Work out the finished part from the listing and answer in its coordinate system (mm). Face numbers are marked on the shaded views. A direction names the side the tool comes from. Round coordinates to 2 decimals unless told otherwise and drop trailing zeros. Loops run counter-clockwise (first coordinate to the right, second up) from the corner with the lowest first, then second, coordinate; pieces in that order, holes last.
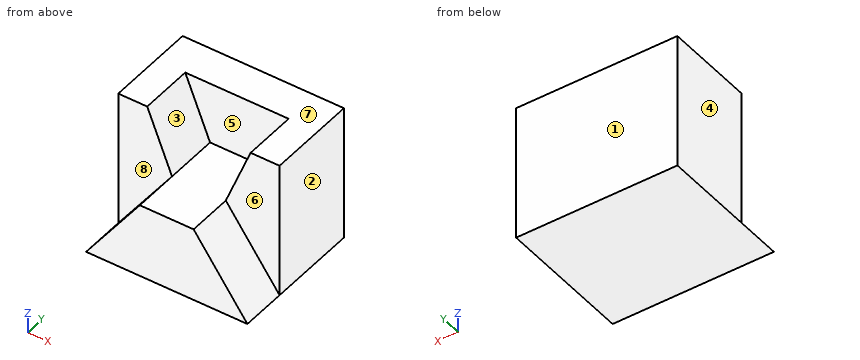
```python
from build123d import *

# Parameters (mm, degrees)
F1_DEPTH = 33
F2_DEPTH = 11
F3_DEPTH = 24


with BuildPart() as f1:
    # F0 (on Front) → F1 (new body)
    with BuildSketch(Plane.XZ):
        Polygon((13, 18), (0, 0), (39, 0), (26, 18), align=None)
        Polygon((0, 33), (0, 0), (13, 18), (7, 33), align=None)
        Polygon((26, 18), (39, 0), (39, 33), (32, 33), align=None)
        Polygon((7, 33), (13, 18), (26, 18), (32, 33), align=None)
    extrude(amount=-F1_DEPTH)

    # F0 (on Front) → F2 (cut)
    with BuildSketch(Plane.XZ):
        Polygon((0, 33), (0, 0), (13, 18), (7, 33), align=None)
        Polygon((7, 33), (13, 18), (26, 18), (32, 33), align=None)
        Polygon((26, 18), (39, 0), (39, 33), (32, 33), align=None)
    extrude(amount=-F2_DEPTH, mode=Mode.SUBTRACT)

    # F0 (on Front) → F3 (cut)
    with BuildSketch(Plane.XZ):
        Polygon((7, 33), (13, 18), (26, 18), (32, 33), align=None)
    extrude(amount=-F3_DEPTH, mode=Mode.SUBTRACT)


solid = f1.part
```
1. Find section C-C (x = 22.5). Write down the section's boundary in (y, z).
Answer key:
outline: (0, 0) - (33, 0) - (33, 33) - (24, 33) - (24, 18) - (0, 18) - close
2. Consider probe 1 along Y at (x, z) = (6, 11); probe 2 along Y at (x, z) = (24.5, 26); probe 3 along X at (y, z) = (23, 23.5). Determine where each line is inside the solid, lowest interval first.
Answer key:
probe 1: y = 11 to 33
probe 2: y = 24 to 33
probe 3: x = 0 to 10.8, 28.2 to 39
3. Determine the mould class of the marked faces 1, 2 and 3 for opening direction X: +X half, -X half, draft (parallel to the pull), parting line (faces both ways), or undercut.
Answer key:
face 1: draft
face 2: +X half
face 3: undercut
4. Find section B-B (y = 16.5). Write down the section's boundary in (x, z).
Answer key:
outline: (0, 0) - (39, 0) - (39, 33) - (32, 33) - (26, 18) - (13, 18) - (7, 33) - (0, 33) - close
5. Which of the six approach directions +Z, -Z, +X, -X, +Y, -Y give full straight-line access (tool end or side, diameter ignored) to the marked faces 4, 5, 6, 7 and 8?
Answer key:
face 4: +Z, -Z, -X, +Y, -Y
face 5: +Z, -Y
face 6: +Z, +X, -Y
face 7: +Z, +X, -X, +Y, -Y
face 8: +Z, -X, -Y
6. Find section D-D (y = 9). Write down the section's boundary in (x, z).
Answer key:
outline: (0, 0) - (39, 0) - (26, 18) - (13, 18) - close
7. Given pin 1 (4 mm diameter, centred on x = 25.5, y = 5, fed in from -Z); pin 2 (10.5 mm diameter, centred on x = 6, z = 23, fed in from -Y); pin 3 (16.5 mm diameter, centred on x = 19.5, z = 28, fed in from -Y); pin 4 (10.5 mm diameter, centred on x = 19.5, y = 10, fed in from +Z), each flat-ended and moving along its own axis, determine where each tip first touches the part or whether it passes through.
Answer key:
pin 1: stops at z = 0
pin 2: stops at y = 11
pin 3: stops at y = 24
pin 4: stops at z = 18
8. Find section A-A (z = 25). Write down the section's boundary in (x, y), then the cut area to 3 significant figures.
Answer key:
outline: (0, 11) - (10.2, 11) - (10.2, 24) - (28.8, 24) - (28.8, 11) - (39, 11) - (39, 33) - (0, 33) - close
area: 616 mm2
